```python
from build123d import *

# Parameters (mm, degrees)
F1_ANGLE = 302.187437


with BuildPart() as f1:
    # F0 (on Front) → F1 (revolve)
    with BuildSketch(Plane.XZ):
        Polygon((-59.469521, 0), (0, 0), (0, 61.875202), (-23.531104, 61.875202), (-23.531104, 27.541725), (-59.469521, 27.541725), align=None)
    revolve(axis=Axis((-29.734761, 0, 0), (-1, 0, 0)), revolution_arc=F1_ANGLE)


solid = f1.part
```
The listing builds one solid part. Answer for the finished solid, in the listing's coordinates (mm). A direction names the side the tool comes from. Coordinates: 2 decimals unless noted, no trailing zeros. Loops run counter-clockwise (first coordinate to the right, second up) from the corner with the lowest first, then second, coordinate; pieces in that order, holes last. Notation, with made-up numbers: (75.25, -17) -> (126.25, -17) arc R16 ccw to (126.25, -12) -> close; hole circle Ø5 at (-28.75, 45). An arc over 180 degrees is marked (long way). Return JSON: item names as keys, results as strings. Group by question number.
(1) A cutting plane is placed at A-A on z = 20. Write down the section's boundary in (x, y), and give its area (3 significant figures).
(2) A cutting plane is placed at D-D on y = -14. Write down the section's boundary in (x, z).
(3) Determine the mould class of faces 1 (the flat face through (-23.54, -20.73, 13.05)), 2 (the flat face through (-23.531, 1, -28)), 3 (the cylindrical face through (-11.93, 31.888, -53.025)) for opening direction Y: released by +Y, released by -Y, zero draft, split by the parting line, or undercut.
(4) A cutting plane is placed at C-C on z = -17. Write down the section's boundary in (x, y).
(5) Given pin 1 Ø8 at (x, z) = (-46, 16) entering from -Y; pin 2 Ø18 at (x, z) = (-16.5, 44.5) entering from -Y; pin 3 Ø6 at (x, z) = (-14, 34) entering from -Y, each flat-ended and moving along its own axis, determine where each tip first touches the part or whether it passes through.
(6) Find the intervals of material crossed by probe 1 along X at (y, z) = (26.5, 29); probe 2 along Y at (x, z) = (-11.5, 15); probe 3 along Y at (x, z) = (-20.5, 40.5), in increasing order. Write a range as from..to.
(7) A cutting plane is placed at B-B on x = -5.5. Write down the section's boundary in (y, z), and give its area (3 significant figures).
(8) Which of the six approach directions +Z, -Z, +X, -X, +Y, -Y give full straight-line access (tool end or side, diameter ignored) to faces 4 (the cylindrical face through (-41.8, 14.2, -23.6)), 5 (the flat face through (0, 1, 1)), 6 (the flat face through (-24, 0, 24))?
The answers:
{
 "1": {"outline": "(-59.47, 0) -> (0, 0) -> (0, 58.55) -> (-23.53, 58.55) -> (-23.53, 18.94) -> (-59.47, 18.94) -> close; (-23.53, -58.55) -> (0, -58.55) -> (0, -31.77) -> (-23.53, -31.77) -> close", "area": "2,690 mm^2"},
 "2": {"outline": "(-59.47, -23.72) -> (-23.53, -23.72) -> (-23.53, -60.27) -> (0, -60.27) -> (0, 8.81) -> (-59.47, 8.81) -> close"},
 "3": {"face 1": "undercut", "face 2": "zero draft", "face 3": "split by the parting line"},
 "4": {"outline": "(-59.47, -21.67) -> (-23.53, -21.67) -> (-23.53, -59.49) -> (0, -59.49) -> (0, 59.49) -> (-23.53, 59.49) -> (-23.53, 21.67) -> (-59.47, 21.67) -> close"},
 "5": {"pin 1": "stops at y = -24.79", "pin 2": "stops at y = 0", "pin 3": "stops at y = -53.55"},
 "6": {"probe 1": "x = -23.53..0", "probe 2": "y = -60.03..-23.83, 0..60.03", "probe 3": "y = 0..46.78"},
 "7": {"outline": "(-52.37, 32.96) arc R61.88 ccw (long way) to (0, 61.88) -> (0, 0) -> close", "area": "10,100 mm^2"},
 "8": {"face 4": "-X", "face 5": "+Z, -Z, +X, +Y, -Y", "face 6": "+Z, +X, -X"}
}
